Autodesk Inventor part; units mm, degrees
ref_plane "YZ Plane" through (0, 0, 0) normal (1, 0, 0) x (0, 1, 0)
ref_plane "XZ Plane" through (0, 0, 0) normal (0, 1, 0) x (-1, 0, 0)
ref_plane "XY Plane" through (0, 0, 0) normal (0, 0, 1) x (1, 0, 0)
sketch "スケッチ1" plane through (0, 0, 0) normal (0, 0, 1) x (1, 0, 0)
  circle A0 centre (0, 0) radius 3.5
  line L0 (3.5, -2.0207) -> (0, -4.0415)
  line L1 (0, -4.0415) -> (-3.5, -2.0207)
  line L2 (-3.5, -2.0207) -> (-3.5, 2.0207)
  line L3 (-3.5, 2.0207) -> (0, 4.0415)
  line L4 (0, 4.0415) -> (3.5, 2.0207)
  line L5 (3.5, 2.0207) -> (3.5, -2.0207)
  point P0 (3.5, 0)
  dimension "d0" = 7
extrude "押し出し1" add sketch "スケッチ1" along normal blind 80
sketch "スケッチ2" plane through (0, 0, 80) normal (0, 0, 1) x (1, 0, 0)
  circle A0 centre (0, 0) radius 2.5
  dimension "d3" = 5
sketch "スケッチ3" plane through (0, 0, 0) normal (0, 0, -1) x (-1, 0, 0)
  circle A0 centre (0, 0) radius 2.5
  dimension "d6" = 5
extrude "押し出し3" cut sketch "スケッチ3" against normal blind 12
extrude "押し出し4" add sketch "スケッチ2" along normal blind 10
thread "ねじ1"
properties part number "六角支柱" material "鉄、ダクタイル鋳鉄"
Part model, mm, in its own coordinate system. A direction names the side the tool comes from. Coordinates: 2 decimals unless noted, no trailing zeros. Loops run counter-clockwise (first coordinate to the right, second up) from the corner with the lowest first, then second, coordinate; pieces in that order, holes last. Notation, with made-up numbers: (37.25, 30) -> (74.25, 30) arc R24 cw to (74.25, 65) -> close; hole circle Ø10 at (86, 17.5). An arc over 180 degrees is marked (long way). Use a Markdown table: item, result. Add a question column.
Item 1: Probe probe 1 along Y at (x, z) = (0, 3.5); probe 2 along Z at (x, y) = (2.25, 2.25); probe 3 along Z at (x, y) = (-1.25, -0.25). List the from-to ranges inside material, lowest first.
Item 2: Band-saw the part on A-A on y = 0. Write the cut outline in (x, z).
Item 3: Band-saw the part on B-B on x = 0.75. Write the cut outline in (y, z).
Item 4: Pull direction X, two halves, no side cores. Call faces 4 (the flat face through (-1.726, -3.045, 39.44)), 5 (the flat face through (0, 0, 12)), 6 (the flat face through (0, 0, 90)): +X half, -X half, draft (parallel to the pull), parting line (faces both ways), or undercut.
Item 5: Which spindle directions (+Z, -Z, +X, -X, +Y, -Y) get a long thin tool onto all of the face, cutting with end or side? Do faces 1 (the flat face through (1.726, 3.045, 39.44)), 2 (the cylindrical face through (-0.54, 2.44, 84.93)), 3 (the cylindrical face through (0.54, -2.44, 5.92)). Say none if no direction does.
Item 6: Flat gauge pins, fed straight in: P1, Ø3, axis at x = -2, z = 77.5, coming from the +Y side; P2, Ø1.5, axis at x = -0.5, y = 0, coming from the -Z side; P3, Ø2, axis at x = -3, y = 2.5, coming from the +Z side. Where does each tip first touch, or does it go through?
Item 7: Band-saw the part on C-C on z = 67. Write the cut outline in (x, y).
Geometry says:
| question | item | result |
|---|---|---|
| 1 | probe 1 | -4.04 to -2.5, 2.5 to 4.04 |
| 1 | probe 2 | 0 to 80 |
| 1 | probe 3 | 12 to 90 |
| 2 | outline | (-3.5, 0) -> (-2.5, 0) -> (-2.5, 12) -> (2.5, 12) -> (2.5, 0) -> (3.5, 0) -> (3.5, 80) -> (2.5, 80) -> (2.5, 90) -> (-2.5, 90) -> (-2.5, 80) -> (-3.5, 80) -> close |
| 3 | outline | (-3.61, 0) -> (-2.38, 0) -> (-2.38, 12) -> (2.38, 12) -> (2.38, 0) -> (3.61, 0) -> (3.61, 80) -> (2.38, 80) -> (2.38, 90) -> (-2.38, 90) -> (-2.38, 80) -> (-3.61, 80) -> close |
| 4 | face 4 | -X half |
| 4 | face 5 | undercut |
| 4 | face 6 | draft |
| 5 | face 1 | +Z, -Z, +X, +Y |
| 5 | face 2 | +Z |
| 5 | face 3 | -Z |
| 6 | P1 | y = 3.75 |
| 6 | P2 | z = 12 |
| 6 | P3 | z = 80 |
| 7 | outline | (-3.5, -2.02) -> (0, -4.04) -> (3.5, -2.02) -> (3.5, 2.02) -> (0, 4.04) -> (-3.5, 2.02) -> close |
